Geometry: final body of the model. Coordinates: model frame, mm. Face numbers are marked on the shaded views. A direction names the side the tool comes from. Give positions to 0.01 mm unless a question says otherwise; leave off trailing zeros. Write each loop counter-clockwise with the first axis right and the second up, starting at its lowest first coordinate (ties: lowest second). Pieces come first, ordered by that corner, then holes. Notation, with made-up numbers: M 49.25,39.25 L 77.25,39.25 A12 cw 77.25,50.25 Z; hole C 47,-25.75 d2. An arc over 180 degrees is marked long. Use a Markdown table: item, result. Add a question column.
(1) Cut plane A-A (x = -11). Output: boundary loops of the cut face in (y, z), plus the area to 3 significant figures.
(2) Cut plane B-B (z = 0). Output: boundary loops of the cut face in (x, y).
(3) Cut plane D-D (y = 8). Output: boundary loops of the cut face in (x, z).
(4) Cut plane C-C (y = -4). State how many separate pieces and enclosed holes the cut face has, plus the area to 3 significant figures.
(5) Pin query (flat end, axial travel): pin 1 Ø0.7 at (x, z) = (-11.5, -10.5) entering from +Y; pin 2 Ø3 at (x, z) = (9.88, 11) entering from +Y; pin 3 Ø2.5 at (x, y) = (-1, 9) entering from +Z. Return the tip coordinate at first contact, or that it passes through.
(6) Material intervals for L1, parallel to Z at x = -11, y = -6; L2, parallel to X at y = -5, z = -11; L3, parallel to Y at x = -2.5, z = -7.5, sorted ascending.
(7) Reachability of the marked faces 1 and 2 from +Z, -Z, +X, -X, +Y, -Y: full face, straight path, thin tool, end or side. Return the list, or none.
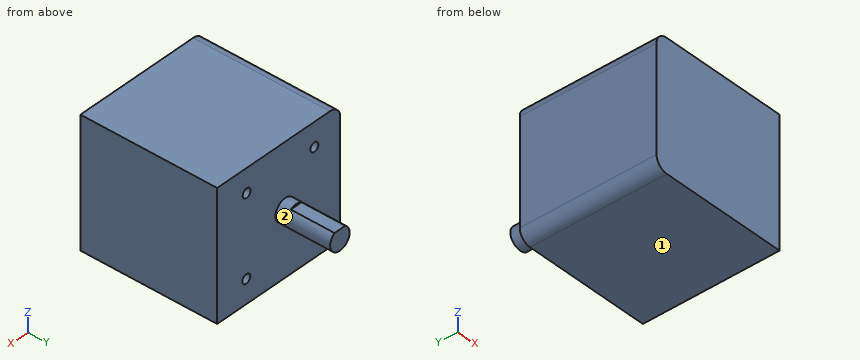
Solid Edge part; units mm, degrees
sketch "Sketch1" plane through (0, 0, 0) normal (0, -1, 0) x (1, 0, 0)
  line L0 (-19, 17.5) -> (19, 17.5)
  line L1 (19, 17.5) -> (19, -17.5)
  line L2 (19, -17.5) -> (-19, -17.5)
  line L3 (-19, -17.5) -> (-19, 17.5)
extrude "Protrusion1" add sketch "Sketch1" along normal blind 37.5
hole "Hole_1" at (10, 0, -11) direction (0, -1, 0) diameter 2.459 depth 10
hole "Hole1" at (-11, 0, 11) direction (0, -1, 0) diameter 2.459 depth 10
hole "Hole2" at (9.8772, 0, 11) direction (0, -1, 0) diameter 2.459 depth 10
hole "Hole3" at (-11, 0, -11) direction (0, -1, 0) diameter 2.459 depth 10
fillet "Round_1" radius 3.175 2 edges at (-19, -18.75, -17.5) (-19, -18.75, 17.5)
sketch "Sketch2" plane through (0, 0, 0) normal (0, 1, 0) x (1, 0, 0)
  circle A0 centre (-2, 0) radius 3
extrude "ExtrudedProtrusion_3" add sketch "Sketch2" along normal blind 15
sketch "Sketch3" plane through (-2, 15, 0) normal (0, 1, 0) x (1, 0, 0)
  line L0 (-1.6583, -2.5) -> (1.6583, -2.5)
  arc A0 (1.6583, -2.5) -> (-1.6583, -2.5) centre (0, 0) cw
extrude "ExtrudedCutout_1" cut sketch "Sketch3" against normal blind 12
Answer list:
| question | item | result |
|---|---|---|
| 1 | outline | M -37.5,-17.5 L 0,-17.5 L 0,-12.23 L -10,-12.23 L -10,-9.77 L 0,-9.77 L 0,9.77 L -10,9.77 L -10,12.23 L 0,12.23 L 0,17.5 L -37.5,17.5 Z |
| 1 | area | 1,260 mm² |
| 2 | outline | M -19,-37.5 L 19,-37.5 L 19,0 L 1,0 L 1,15 L -5,15 L -5,0 L -19,0 Z |
| 3 | outline | M -3.66,2.5 A3 ccw long -0.34,2.5 Z |
| 4 | separate pieces | 1 |
| 4 | enclosed holes | 4 |
| 4 | area | 1,310 mm² |
| 5 | pin 1 | y = -10 |
| 5 | pin 2 | y = 0 |
| 5 | pin 3 | z = 2.5 |
| 6 | L1 | -17.5 to -12.23, -9.77 to 9.77, 12.23 to 17.5 |
| 6 | L2 | -19 to -12.23, -9.77 to 8.77, 11.23 to 19 |
| 6 | L3 | -37.5 to 0 |
| 7 | face 1 | -Z, +X, -X, +Y, -Y |
| 7 | face 2 | +Y |
